Read the model definition and answer for the solid it produces. Units are mm, in the model's axes. Give positions to 0.01 mm unless a question says otherwise; leave off trailing zeros. Write each loop counter-clockwise with the first axis right and the second up, starting at its lowest first coordinate (ties: lowest second). Pieces come first, ordered by that corner, then holes. Notation, with made-up numbers: (85.25, 64.25) -> (109.25, 64.25) arc R18 ccw to (109.25, 97.25) -> close; hole circle Ø2 at (4.5, 25). An arc over 180 degrees is marked (long way). Write item = value, one per line.
from build123d import *

# Parameters (mm, degrees)
ESQUISSE1_W               = 110
ESQUISSE1_H               = 130
T_LE_DE_BASE_PLI_E1_DEPTH = 0.7366
D_GAGEMENT_M51_D          = 5.5
COIN_BRIS_1_START         = -0.7366
COIN_BRIS_1_DEPTH         = 0.7366


# Read off the part's stored shape, not the designer's step: Coin-brisé1
# Sheet-metal steps are written as plain solids
with BuildPart() as part:
    # Esquisse1 → Tôle de base pliée1 (new body)
    with BuildSketch(Plane.XY):
        Rectangle(ESQUISSE1_W, ESQUISSE1_H)
    extrude(amount=-T_LE_DE_BASE_PLI_E1_DEPTH)

    # Dégagement M51 (through all)
    with Locations(Plane.XY):
        with Locations((-45, 47.5), (45, 47.5), (45, -47.5), (-45, -47.5)):
            Hole(D_GAGEMENT_M51_D / 2)

    # Coin-brisé1 outline → Coin-brisé1 (cut)
    with BuildSketch(Plane.XY.offset(COIN_BRIS_1_START)):
        with BuildLine():
            ThreePointArc((55, -63), (54.414213562, -64.414213562), (53, -65))
            Line((53, -65), (55, -65))
            Line((55, -65), (55, -63))
        make_face()
        with BuildLine():
            Line((-55, -65), (-53, -65))
            ThreePointArc((-53, -65), (-54.414213562, -64.414213562), (-55, -63))
            Line((-55, -63), (-55, -65))
        make_face()
        with BuildLine():
            ThreePointArc((53, 65), (54.414213562, 64.414213562), (55, 63))
            Line((55, 63), (55, 65))
            Line((55, 65), (53, 65))
        make_face()
        with BuildLine():
            Line((-55, 65), (-55, 63))
            ThreePointArc((-55, 63), (-54.414213562, 64.414213562), (-53, 65))
            Line((-53, 65), (-55, 65))
        make_face()
    extrude(amount=COIN_BRIS_1_DEPTH, mode=Mode.SUBTRACT)


solid = part.part
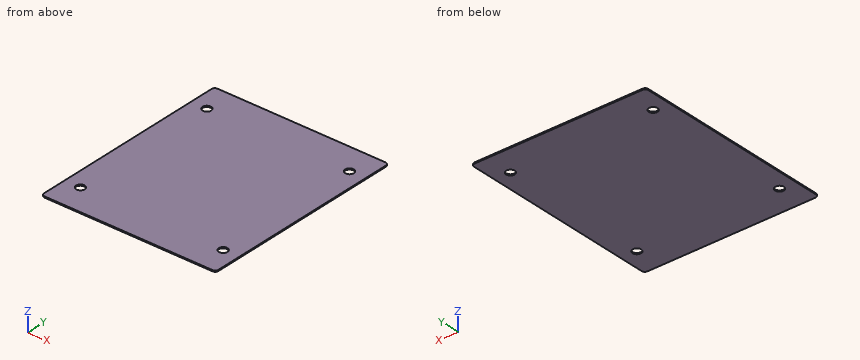
(1) The part is cut by section A-A on x = -45. Determine the outline of the cut face in (y, z).
Checks:
outline = (-65, -0.74) -> (-50.25, -0.74) -> (-50.25, 0) -> (-65, 0) -> close; (-44.75, -0.74) -> (44.75, -0.74) -> (44.75, 0) -> (-44.75, 0) -> close; (50.25, -0.74) -> (65, -0.74) -> (65, 0) -> (50.25, 0) -> close
(2) Consider L1, parallel to Y at x = 45, z = -0.2; L2, parallel to Y at x = 44, z = -0.5; L3, parallel to X at y = 47, z = -0.55. Determine where each line is inside the solid, lowest interval first.
Checks:
L1 = -65 to -50.25, -44.75 to 44.75, 50.25 to 65
L2 = -65 to -50.06, -44.94 to 44.94, 50.06 to 65
L3 = -55 to -47.7, -42.3 to 42.3, 47.7 to 55
(3) The part is cut by section B-B on y = 47.5. Determine the outline of the cut face in (x, z).
Checks:
outline = (-55, -0.74) -> (-47.75, -0.74) -> (-47.75, 0) -> (-55, 0) -> close; (-42.25, -0.74) -> (42.25, -0.74) -> (42.25, 0) -> (-42.25, 0) -> close; (47.75, -0.74) -> (55, -0.74) -> (55, 0) -> (47.75, 0) -> close
